For this review, take the finished solid that the model builds, in its own axes (mm). Round coordinates to 2 decimals unless told otherwise and drop trailing zeros. Order: outer loops, then holes, each group sorted by start corner. A loop starts at its lowest first (then second) coordinate and runs counter-clockwise, first axis right, second up. Notation, with made-up numbers: M 79,17.5 L 121,17.5 A28 ccw 121,44.5 Z; hole C 74,88.25 d3. An arc over 180 degrees is marked long. Write item = value, one per line. Start each with the question number.
from build123d import *

# Parameters (mm, degrees)
F0_R     = 6.35
F1_DEPTH = 6.35


with BuildPart() as f1:
    # F0 (on Front) → F1 (new body)
    with BuildSketch(Plane.XZ):
        with BuildLine():
            ThreePointArc((689.715387, -21.48571), (724.74821, -13.547113), (716.809613, 21.48571))
            ThreePointArc((716.809613, 21.48571), (351.63125, 127), (-13.547113, 21.48571))
            ThreePointArc((-13.547113, 21.48571), (-21.48571, -13.547113), (13.547113, -21.48571))
            ThreePointArc((13.547113, -21.48571), (351.63125, 76.2), (689.715387, -21.48571))
        make_face()
        Circle(F0_R, mode=Mode.SUBTRACT)
        with Locations((64.770503, 35.920821)):
            Circle(F0_R, mode=Mode.SUBTRACT)
        with Locations((703.2625, 0)):
            Circle(F0_R, mode=Mode.SUBTRACT)
        with Locations((638.491997, 35.920821)):
            Circle(F0_R, mode=Mode.SUBTRACT)
        with Locations((133.16127, 64.350144)):
            Circle(F0_R, mode=Mode.SUBTRACT)
        with Locations((204.309192, 84.929181)):
            Circle(F0_R, mode=Mode.SUBTRACT)
        with Locations((277.316359, 97.398219)):
            Circle(F0_R, mode=Mode.SUBTRACT)
        with Locations((351.63125, 101.6)):
            Circle(F0_R, mode=Mode.SUBTRACT)
        with Locations((498.953308, 84.929181)):
            Circle(F0_R, mode=Mode.SUBTRACT)
        with Locations((570.10123, 64.350144)):
            Circle(F0_R, mode=Mode.SUBTRACT)
        with Locations((425.946141, 97.398219)):
            Circle(F0_R, mode=Mode.SUBTRACT)
    extrude(amount=F1_DEPTH)


solid = f1.part
(1) We need section A-A, the plane x = 0. Write out the cut boundary in (y, z), then the cut area to 3 significant figures.
(2) Draft analysis for pull direction X (two halves, no side actions). For faces 1 (the cylindrical face through (357.02, -3.13, 126.98)), 2 (the cylindrical face through (-1.38, -3.13, -6.2)), 3 (the flat face through (350, -6.35, 91)), 4 (the cylindrical face through (424.57, -3.13, 91.2)), state which applies: released by +X, released by -X, zero draft, split by the parting line, or undercut.
(3) We need section B-B, the plane y = -1.25. State how many separate pieces and enclosed holes the cut face has, then the cut area to 3 significant figures.
(4) Insertion check: pin 1 (1 mm diameter, centred on y = -3.5, z = 77, fed in from +X). The pin has a flat end and moves straight along its axis. Give the tip position at first contact, or say it passes through.
(5) We need section D-D, the plane x = 393.5. Write out the cut boundary in (y, z).
(6) For line 1 along X through (y, z) = (-4.25, -7); line 2 along Z through (x, y) = (275.5, -5); line 3 along X through (y, z) = (-3, 20), list the stretches that pass through material, from the lowest coordinate up.
(7) We need section C-C, the plane z = 0. Write out the cut boundary in (x, y).
Values:
q1.outline = M -6.35,-25.4 L 0,-25.4 L 0,-6.35 L -6.35,-6.35 Z; M -6.35,6.35 L 0,6.35 L 0,29.81 L -6.35,29.81 Z
q1.area = 270 mm²
q2.face_1 = split by the parting line
q2.face_2 = undercut
q2.face_3 = zero draft
q2.face_4 = undercut
q3.separate_pieces = 1
q3.enclosed_holes = 11
q3.area = 38,300 mm²
q4.pin_1 = 609.71
q5.outline = M -6.35,74.82 L 0,74.82 L 0,125.72 L -6.35,125.72 Z
q6.line_1 = -24.42 to 37.69, 665.57 to 727.68
q6.line_2 = 71.61 to 91.31, 103.48 to 122.75
q6.line_3 = -15.66 to 90.69, 612.57 to 718.92
q7.outline = M -25.4,-6.35 L -6.35,-6.35 L -6.35,0 L -25.4,0 Z; M 6.35,-6.35 L 50.3,-6.35 L 50.3,0 L 6.35,0 Z; M 652.96,-6.35 L 696.91,-6.35 L 696.91,0 L 652.96,0 Z; M 709.61,-6.35 L 728.66,-6.35 L 728.66,0 L 709.61,0 Z
